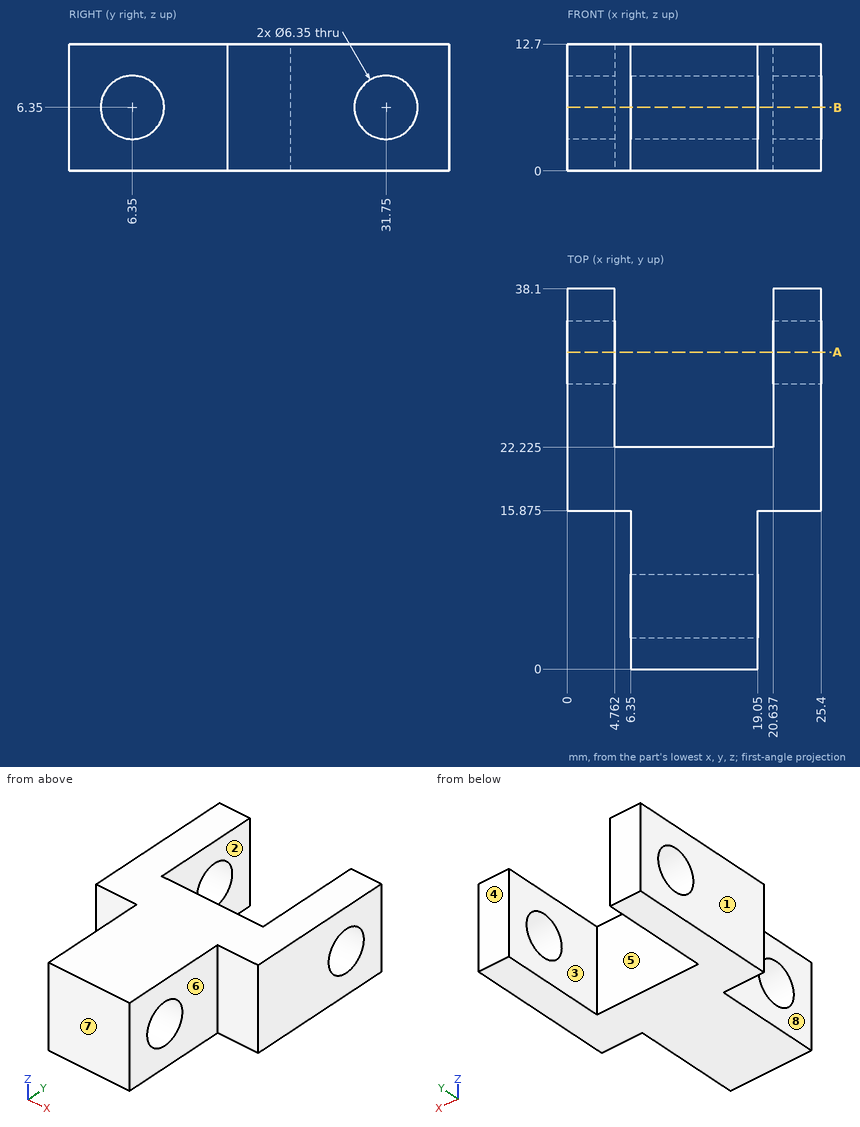
The drawing under review shows one solid part. Ordinate dimensions are in mm from its lowest x, y, z. A direction names the side the tool comes from. Coordinates: 2 decimals unless noted, no trailing zeros. Order: outer loops, then holes, each group sorted by start corner. A loop starts at its lowest first (then second) coordinate and runs counter-clockwise, first axis right, second up. Notation, with made-up numbers: (47.5, 27.5) -> (71.5, 27.5) arc R21 cw to (71.5, 48.5) -> close; hole circle Ø3 at (75, 14). An arc over 180 degrees is marked (long way). One line per item, written item: value.
1) To check wall thickness, follow probe 1 along X at (y, z) = (25.5, 6.25); probe 2 along Y at (x, z) = (12, 6.5) (1 decimal); probe 3 along X at (y, z) = (9, 8.5). State the ranges of each line that lie inside material, in increasing order. Write a range as [from, to].
Output values:
probe 1: x = [0, 4.76], [20.64, 25.4]
probe 2: y = [0, 3.2], [9.5, 22.2]
probe 3: x = [6.35, 19.05]
2) Machinability: for the marked faces 5, 6, 7 and 8, which of the approach directions +Z, -Z, +X, -X, +Y, -Y give a long, thin tool a straight path to every point of the face, cutting with its end or side? Answer none if there is none.
Output values:
face 5: +Z, -Z, +Y
face 6: +Z, -Z, +X, -Y
face 7: +Z, -Z, +X, -X, -Y
face 8: +Z, -Z, -X, -Y
3) We need section A-A, the plane y = 31.75. Give the boundary of the cut face in (x, z) (1 decimal).
Output values:
outline: (0, 0) -> (4.8, 0) -> (4.8, 3.2) -> (0, 3.2) -> close; (0, 9.5) -> (4.8, 9.5) -> (4.8, 12.7) -> (0, 12.7) -> close; (20.6, 0) -> (25.4, 0) -> (25.4, 3.2) -> (20.6, 3.2) -> close; (20.6, 9.5) -> (25.4, 9.5) -> (25.4, 12.7) -> (20.6, 12.7) -> close
4) Clearance check with flat-ended pins moving along their axes: P1, Ø4, axis at y = 8, z = 9, coming from the +X side; P2, Ø5.5, axis at y = 31.75, z = 6.35, coming from the +X side; P3, Ø4, axis at x = 13.5, z = 8.5, coming from the +Y side (1 decimal); P4, Ø3, axis at x = 2, z = 6.5, coming from the -Y side (1 decimal). State where each tip first meets the part, or that it passes through.
Output values:
P1: stops at x = 19.05
P2: passes through
P3: stops at y = 22.2
P4: stops at y = 15.9
5) We need section B-B, the plane z = 6.35. Count the separate pieces of the cut face and the enclosed holes in it, then the cut area to 3 significant figures.
Output values:
separate pieces: 4
enclosed holes: 0
area: 373 mm2
6) Draft analysis for pull direction X (two halves, no side actions). For the marked faces 1, 2, 3 and 4, state which applies: +X half, -X half, draft (parallel to the pull), parting line (faces both ways), or undercut.
Output values:
face 1: -X half
face 2: undercut
face 3: undercut
face 4: draft
